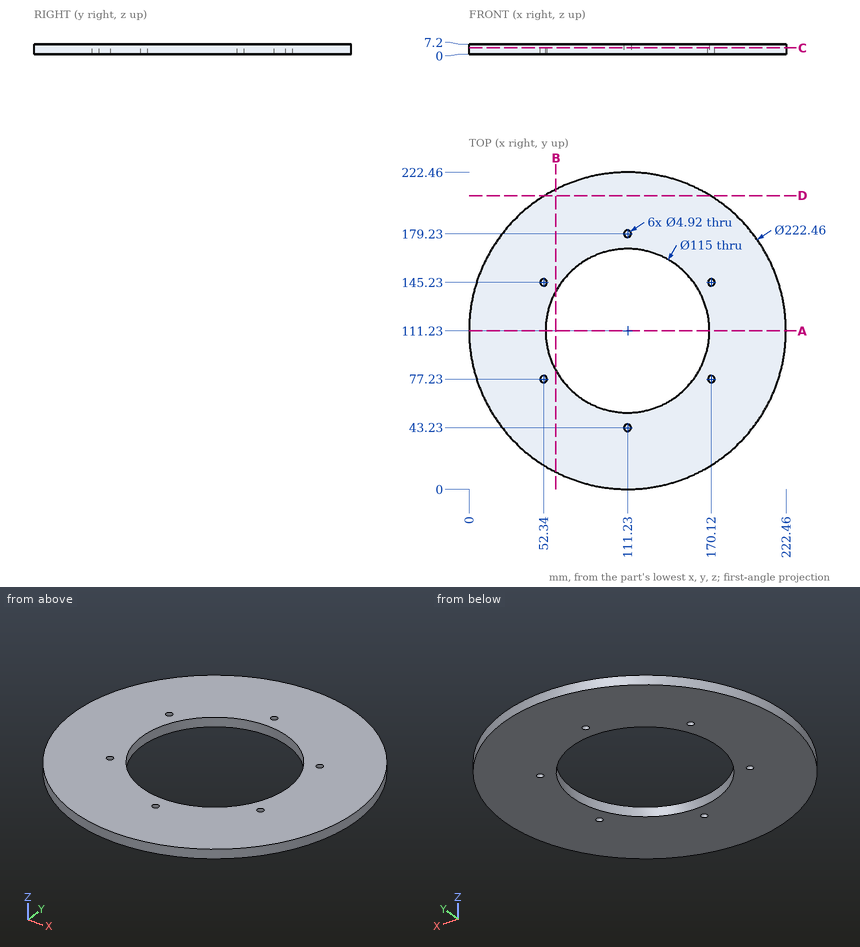
Source: three-view drawing plus pictorial views. Frame: mm from the lowest corner of the part. Round coordinates to 2 decimals unless told otherwise and drop trailing zeros. Loops run counter-clockwise (first coordinate to the right, second up) from the corner with the lowest first, then second, coordinate; pieces in that order, holes last. Notation, with made-up numbers: (73, -12.5) - (89, -12.5) arc R31 cw to (89, 19.5) - close; hole circle Ø6 at (-37, 5). An arc over 180 degrees is marked (long way). Write each question's results on one line, items separated by ' | '. Start each with the question number.
1) Cut plane A-A on y = 111.23. Return loops of the section in (x, z), then the cut area to 3 significant figures.
2) First-contact query: P1, Ø1.5, axis at y = 177.5, z = 5.5, coming from the -X side (1 decimal); P2, Ø1.5, axis at x = 50, z = 4.5, coming from the +Y side; P3, Ø1.5, axis at y = 157.5, z = 4, coming from the -X side. Flat tips, straight axial feed; report the tip coordinate or a pass-through.
3) Cut plane D-D on y = 206. Return loops of the section in (x, z).
4) Cut plane C-C on z = 4.5. Return loops of the section in (x, y).
5) Cut plane B-B on x = 61. Return loops of the section in (y, z).
6) Line query: probe 1 along Y at (x, z) = (111.23, 2); probe 2 along X at (y, z) = (100.5, 4.5); probe 3 along X at (y, z) = (61, 6.25) (1 decimal). Output: solid intervals per line, ascending. Write a range as [from, to].
Verdict:
1) outline: (0, 0) - (53.73, 0) - (53.73, 7.2) - (0, 7.2) - close; (168.73, 0) - (222.46, 0) - (222.46, 7.2) - (168.73, 7.2) - close | area: 774 mm2
2) P1: stops at x = 21.3 | P2: stops at y = 204.58 | P3: stops at x = 9.74
3) outline: (53, 0) - (169.46, 0) - (169.46, 7.2) - (53, 7.2) - close
4) outline: circle Ø222.46 at (111.23, 111.23); hole circle Ø4.92 at (52.34, 77.23); hole circle Ø4.92 at (52.34, 145.23); hole circle Ø115 at (111.23, 111.23); hole circle Ø4.92 at (111.23, 43.23); hole circle Ø4.92 at (111.23, 179.23); hole circle Ø4.92 at (170.12, 77.23); hole circle Ø4.92 at (170.12, 145.23)
5) outline: (11.99, 0) - (83.24, 0) - (83.24, 7.2) - (11.99, 7.2) - close; (139.22, 0) - (210.47, 0) - (210.47, 7.2) - (139.22, 7.2) - close
6) probe 1: y = [0, 40.77], [45.69, 53.73], [168.73, 176.77], [181.69, 222.46] | probe 2: x = [0.52, 54.74], [167.72, 221.94] | probe 3: x = [12, 83.2], [139.2, 210.5]
